from build123d import *

# Parameters (mm, degrees)
SZKIC1_R                    = 2
DODANIE_WYCI_GNI_CIE1_DEPTH = 5
ZAOKR_GLENIE1_R             = 2
ZAOKR_GLENIE2_R             = 8


with BuildPart() as part:
    # Szkic1 → Dodanie-wyciągnięcie1 (new body)
    with BuildSketch(Plane.XY):
        with BuildLine():
            ThreePointArc((12, 0), (15, 3), (18, 0))
            Line((18, 0), (18, -17.5))
            Line((18, -17.5), (28, -17.5))
            Line((28, -17.5), (28, 17.5))
            Line((28, 17.5), (2, 17.5))
            Line((2, 17.5), (-2, 17.5))
            Line((-2, 17.5), (-28, 17.5))
            Line((-28, 17.5), (-28, -17.5))
            Line((-28, -17.5), (-18, -17.5))
            Line((-18, -17.5), (-18, 0))
            ThreePointArc((-18, 0), (-15, 3), (-12, 0))
            Line((-12, 0), (-12, -17.5))
            Line((-12, -17.5), (12, -17.5))
            Line((12, -17.5), (12, 0))
        make_face()
        with BuildLine():
            Line((-2, 17.5), (2, 17.5))
            Line((2, 17.5), (2, 22.5))
            ThreePointArc((2, 22.5), (0, 20.5), (-2, 22.5))
            Line((-2, 22.5), (-2, 17.5))
        make_face()
        with Locations((0, 22.5)):
            Circle(SZKIC1_R)
    extrude(amount=DODANIE_WYCI_GNI_CIE1_DEPTH)

    # Zaokrąglenie1
    zaokr_glenie1_edges = [part.edges().sort_by_distance(p)[0] for p in [
        (12, -17.5, 2.5),
        (-12, -17.5, 2.5),
        (-18, -17.5, 2.5),
        (-28, -17.5, 2.5),
        (-2, 17.5, 2.5),
        (2, 17.5, 2.5),
        (28, -17.5, 2.5),
        (18, -17.5, 2.5),
    ]]
    fillet(zaokr_glenie1_edges, radius=ZAOKR_GLENIE1_R)

    # Zaokrąglenie2
    zaokr_glenie2_edges = [part.edges().sort_by_distance(p)[0] for p in [
        (-28, 17.5, 2.5),
        (28, 17.5, 2.5),
    ]]
    fillet(zaokr_glenie2_edges, radius=ZAOKR_GLENIE2_R)


solid = part.part
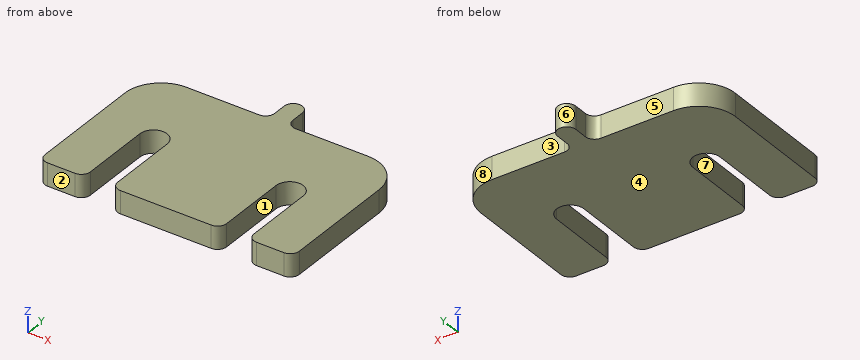
Build history of the part. All positions in model axes, mm. Face numbers are marked on the shaded views. A direction names the side the tool comes from. Give positions to 0.01 mm unless a question says otherwise; leave off trailing zeros. Loops run counter-clockwise (first coordinate to the right, second up) from the corner with the lowest first, then second, coordinate; pieces in that order, holes last. Notation, with made-up numbers: (12.5, 43) - (24.5, 43) arc R20 cw to (24.5, 82) - close; hole circle Ø4 at (-10, -23.75). An arc over 180 degrees is marked (long way). Write item = value, one per line. Start each with the question number.
1) Pull direction X, two halves, no side cores. Call the marked faces 6, 7 and 8: +X half, -X half, draft (parallel to the pull), parting line (faces both ways), or undercut.
2) Band-saw the part on D-D on x = 15. Give the cut face in (y, z).
3) Drop flat-ended pins along their axis: pin 1 Ø0.9 at (y, z) = (21, 2) entering from -X; pin 2 Ø1.5 at (x, z) = (-8.5, 2.5) entering from +Y. Give the stop position or say it passes through.
4) Tool access for the marked faces 1, 2, 3, 4 and 5: list every direction of +Z, -Z, +X, -X, +Y, -Y with a clear straight run to the whole face (end or side of a thin tool).
5) Band-saw the part on B-B on z = 1.6. Give the cut face in (x, y).
6) Band-saw the part on C-C on x = 9. Give the cut face in (y, z), plus the area to 3 significant figures.
7) Probe probe 1 along X at (y, z) = (-8.5, 1.65); probe 2 along X at (y, z) = (1, 4.3); probe 3 along Y at (x, z) = (-8.5, 4.65). List the from-to ranges inside material, lowest first. Write a range as from..to.
8) Band-saw the part on A-A on y = -2. Give the cut face in (x, z).
Final values:
q1.face_6 = parting line
q1.face_7 = undercut
q1.face_8 = +X half
q2.outline = (3, 0) - (17.5, 0) - (17.5, 5) - (3, 5) - close
q3.pin_1 = -2
q3.pin_2 = 17.5
q4.face_1 = +Z, -Z, -Y
q4.face_2 = +Z, -Z, +X, -X, -Y
q4.face_3 = +Z, -Z, +X, +Y
q4.face_4 = -Z, +X, -X, +Y, -Y
q4.face_5 = +Z, -Z, -X, +Y
q5.outline = (-28, -15.5) arc R2 ccw to (-26, -17.5) - (-20, -17.5) arc R2 ccw to (-18, -15.5) - (-18, 0) arc R3 cw to (-12, 0) - (-12, -15.5) arc R2 ccw to (-10, -17.5) - (10, -17.5) arc R2 ccw to (12, -15.5) - (12, 0) arc R3 cw to (18, 0) - (18, -15.5) arc R2 ccw to (20, -17.5) - (26, -17.5) arc R2 ccw to (28, -15.5) - (28, 9.5) arc R8 ccw to (20, 17.5) - (4, 17.5) arc R2 cw to (2, 19.5) - (2, 22.5) arc R2 ccw to (-2, 22.5) - (-2, 19.5) arc R2 cw to (-4, 17.5) - (-20, 17.5) arc R8 ccw to (-28, 9.5) - close
q6.outline = (-17.5, 0) - (17.5, 0) - (17.5, 5) - (-17.5, 5) - close
q6.area = 175 mm²
q7.probe_1 = -28..-18, -12..12, 18..28
q7.probe_2 = -28..-17.83, -12.17..12.17, 17.83..28
q7.probe_3 = -17.5..17.5
q8.outline = (-28, 0) - (-18, 0) - (-18, 5) - (-28, 5) - close; (-12, 0) - (12, 0) - (12, 5) - (-12, 5) - close; (18, 0) - (28, 0) - (28, 5) - (18, 5) - close
